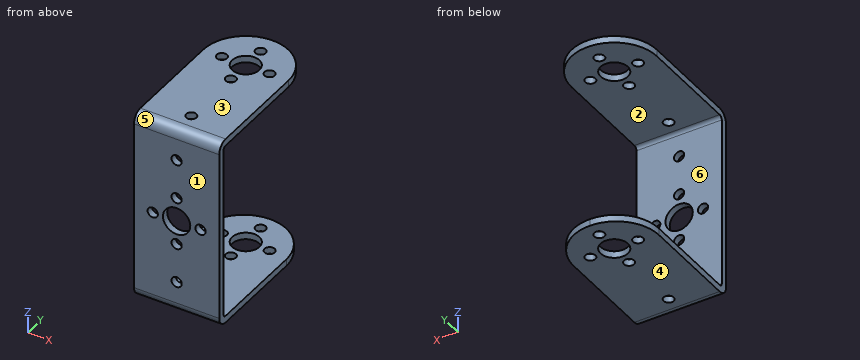
from build123d import *

# Parameters (mm, degrees)
BASE_FLANGE1_DEPTH           = 2
EDGE_FLANGE1_DEPTH           = 25
EDGE_FLANGE2_STRIP_W         = 10
EDGE_FLANGE2_STRIP_H         = 2
EDGE_FLANGE2_STRIP_CUT_DEPTH = 25
EDGE_FLANGE2_DEPTH           = 25
CUT_EXTRUDE1_DEPTH           = 2
SKETCH19_R                   = 4
CUT_EXTRUDE2_DEPTH           = 72.107313267
M3X0_5_TAPPED_HOLE1_D        = 3
SKETCH22_R                   = 4
CUT_EXTRUDE3_DEPTH           = 72.702510416
M3X0_5_TAPPED_HOLE2_D        = 3


# Sheet-metal steps are written as plain solids
with BuildPart() as part:
    # Sketch8 → Base-Flange1 (new body)
    with BuildSketch(Plane.XY):
        with BuildLine():
            Line((-12.5, 0), (12.5, 0))
            Line((12.5, 0), (12.5, 29.5))
            ThreePointArc((12.5, 29.5), (0, 42), (-12.5, 29.5))
            Line((-12.5, 29.5), (-12.5, 0))
        make_face()
    extrude(amount=-BASE_FLANGE1_DEPTH)

    # Edge-Flange1 section (across the edge) → Edge-Flange1 (add)
    with BuildSketch(Plane(origin=(12.5, -1, -2), x_dir=(0, 1, 0), z_dir=(-1, 0, 0))):
        with BuildLine():
            Line((-2, 1), (-2, 52))
            Line((-2, 52), (0, 52))
            Line((0, 52), (0, 1))
            ThreePointArc((0, 1), (0.292893219, 0.292893219), (1, 0))
            Line((1, 0), (1, -2))
            ThreePointArc((1, -2), (-1.121320344, -1.121320344), (-2, 1))
        make_face()
    extrude(amount=EDGE_FLANGE1_DEPTH)

    # Edge-Flange2 strip (across the edge) → Edge-Flange2 strip cut (cut)
    with BuildSketch(Plane(origin=(12.5, -1, -54), x_dir=(0, 0, 1), z_dir=(-1, 0, 0))):
        with Locations((-4, -1)):
            Rectangle(EDGE_FLANGE2_STRIP_W, EDGE_FLANGE2_STRIP_H)
    extrude(amount=EDGE_FLANGE2_STRIP_CUT_DEPTH, mode=Mode.SUBTRACT)

    # Edge-Flange2 section (across the edge) → Edge-Flange2 (add)
    with BuildSketch(Plane(origin=(12.5, -1, -54), x_dir=(0, 0, 1), z_dir=(-1, 0, 0))):
        with BuildLine():
            Line((-2, 1), (-2, 42))
            Line((-2, 42), (0, 42))
            Line((0, 42), (0, 1))
            ThreePointArc((0, 1), (0.292893219, 0.292893219), (1, 0))
            Line((1, 0), (1, -2))
            ThreePointArc((1, -2), (-1.121320344, -1.121320344), (-2, 1))
        make_face()
    extrude(amount=EDGE_FLANGE2_DEPTH)

    # Sketch18 → Cut-Extrude1 (cut)
    with BuildSketch(Plane(origin=(0, 0, -56), x_dir=(-1, 0, 0), z_dir=(0, 0, -1))):
        with BuildLine():
            ThreePointArc((2e-08, 41), (8.838834772, 37.338834758), (12.5, 28.5))
            Line((12.5, 28.5), (12.5, 41))
            Line((12.5, 41), (2e-08, 41))
        make_face()
        with BuildLine():
            ThreePointArc((-12.5, 28.5), (-8.838834758, 37.338834772), (2e-08, 41))
            Line((2e-08, 41), (-12.5, 41))
            Line((-12.5, 41), (-12.5, 28.5))
        make_face()
    extrude(amount=-CUT_EXTRUDE1_DEPTH, mode=Mode.SUBTRACT)

    # Sketch19 → Cut-Extrude2 (cut, through all)
    with BuildSketch(Plane.XY):
        with Locations((0, 29.5)):
            Circle(SKETCH19_R)
    extrude(amount=-CUT_EXTRUDE2_DEPTH, mode=Mode.SUBTRACT)

    # M3x0.5 Tapped Hole1 (through all)
    with Locations(Plane.XY):
        with Locations((0, 36.5), (-7, 29.5), (0, 22.5), (7, 29.5), (0, 3.9), (0, -12.97)):
            Hole(M3X0_5_TAPPED_HOLE1_D / 2)

    # Sketch22 → Cut-Extrude3 (cut, through all)
    with BuildSketch(Plane(origin=(0, -1, 0), x_dir=(1, 0, 0), z_dir=(0, 1, 0))):
        with Locations(Location((0, 28, 0), (0, 0, 270))):
            Circle(SKETCH22_R)
    extrude(amount=-CUT_EXTRUDE3_DEPTH, mode=Mode.SUBTRACT)

    # M3x0.5 Tapped Hole2 (through all)
    with Locations(Plane(origin=(0, -1, 0), x_dir=(1, 0, 0), z_dir=(0, 1, 0))):
        with Locations((7, 28), (-7, 28), (0, 35), (0, 21), (0, 9.4), (0, 46.6)):
            Hole(M3X0_5_TAPPED_HOLE2_D / 2)


solid = part.part
Verification items for the finished model (mm, model axes). Face numbers are marked on the shaded views. A direction names the side the tool comes from. Coordinates: 2 decimals unless noted, no trailing zeros. Order: outer loops, then holes, each group sorted by start corner. A loop starts at its lowest first (then second) coordinate and runs counter-clockwise, first axis right, second up. Notation, with made-up numbers: M 39,82.5 L 52,82.5 A30 cw 52,121.5 Z; hole C 89,-24 d3. An arc over 180 degrees is marked long. Write each question's results on one line, items separated by ' | '.
1) Section check D-D on x = -10. Record the cut outline in (y, z).
Solved:
outline: M -3,-53 A3 ccw 0,-56 L 36,-56 L 36,-54 L 0,-54 A1 cw -1,-53 L -1,-3 A1 cw 0,-2 L 37,-2 L 37,0 L 0,0 A3 ccw -3,-3 Z
2) Release check for a two-part mould opening along Z. For the marked faces 1, 2, 3 and 4 record: pulls with the +Z half, pulls with the -Z half, needs draft (parallel to the pull), parting line crosses it, or undercut.
Solved:
face 1: needs draft | face 2: undercut | face 3: pulls with the +Z half | face 4: pulls with the -Z half
3) Section check A-A on y = 10. Record the cut outline in (x, z), plus the area to 3 significant figures.
Solved:
outline: M -12.5,-56 L 12.5,-56 L 12.5,-54 L -12.5,-54 Z; M -12.5,-2 L 12.5,-2 L 12.5,0 L -12.5,0 Z | area: 100 mm²
4) Section check C-C on x = 7. Record the cut outline in (y, z).
Solved:
outline: M -3,-53 A3 ccw 0,-56 L 28,-56 L 28,-54 L 0,-54 A1 cw -1,-53 L -1,-29.5 L -3,-29.5 Z; M -3,-26.5 L -1,-26.5 L -1,-3 A1 cw 0,-2 L 28,-2 L 28,0 L 0,0 A3 ccw -3,-3 Z; M 31,-56 L 38.86,-56 L 38.86,-54 L 31,-54 Z; M 31,-2 L 39.86,-2 L 39.86,0 L 31,0 Z
5) Section check B-B on z = -35. Record the cut outline in (x, y), plus the area to 3 significant figures.
Solved:
outline: M -12.5,-3 L -1.5,-3 L -1.5,-1 L -12.5,-1 Z; M 1.5,-3 L 12.5,-3 L 12.5,-1 L 1.5,-1 Z | area: 44.0 mm²
6) Access from +Z, -Z, +X, -X, +Y, -Y to the whole of each face (thin tool, end or side, straight path). Record for the marked faces 5 and 6.
Solved:
face 5: +Z, +X, -X, -Y | face 6: +X, -X, +Y
7) Gauge pin test, flat ends, axial feed: pin 1 Ø3.5 at (x, z) = (7, -28) entering from +Y; pin 2 Ø1.8 at (x, y) = (7, 29.5) entering from +Z. Record the tip position at first contact, or that the pin passes through.
Solved:
pin 1: stops at y = -1 | pin 2: passes through
8) Scan lines: line 1 along Z through (x, y) = (7.25, 2.5); line 2 along Y through (x, z) = (0, -54.75); line 3 along Y through (x, z) = (-2.25, -44). Record each from-to range of solid material in increasing order. Write a range as [from, to].
Solved:
line 1: z = [-56, -54], [-2, 0] | line 2: y = [-2.44, 2.4], [5.4, 21], [24, 25.5], [33.5, 35], [38, 41] | line 3: y = [-3, -1]
